Can you work these out from the drawing? Everything is in mm from the part's minimum corner. A direction names the side the tool comes from. Give positions to 0.01 mm unless a question says otherwise; leave off trailing zeros. Loops run counter-clockwise (first coordinate to the right, second up) from the corner with the lowest first, then second, coordinate; pieces in that order, holes last.
Q1. If we section it at A-A (y = 5.5): Please give me the cut outline in (x, z).
Q2. Will these pins go through, and if not, where does the flat tip stop? P1, Ø1.5, axis at x = 1.5, z = 4, coming from the -Y side; P2, Ø1, axis at y = 2, z = 7, coming from the +X side (1 decimal).
Q3. If we section it at C-C (x = 0.8): Please give me the cut outline in (y, z).
Q4. I need wall thicknesses on line 1 (Z direction, x = 2.05, y = 4.5); line 2 (X direction, y = 3.25, z = 11.25); line 3 (Y direction, x = 1.55, z = 5.5) (1 decimal). Which ranges of each line are inside material? Lowest first, please.
Q5. If we section it at B-B (z = 6.25): Please give me the cut outline in (x, y).
Q6. For the marked faces 1 and 2, which set-ups out of +Z, -Z, +X, -X, +Y, -Y let a thin tool reach every point of the face, with its end or its side?
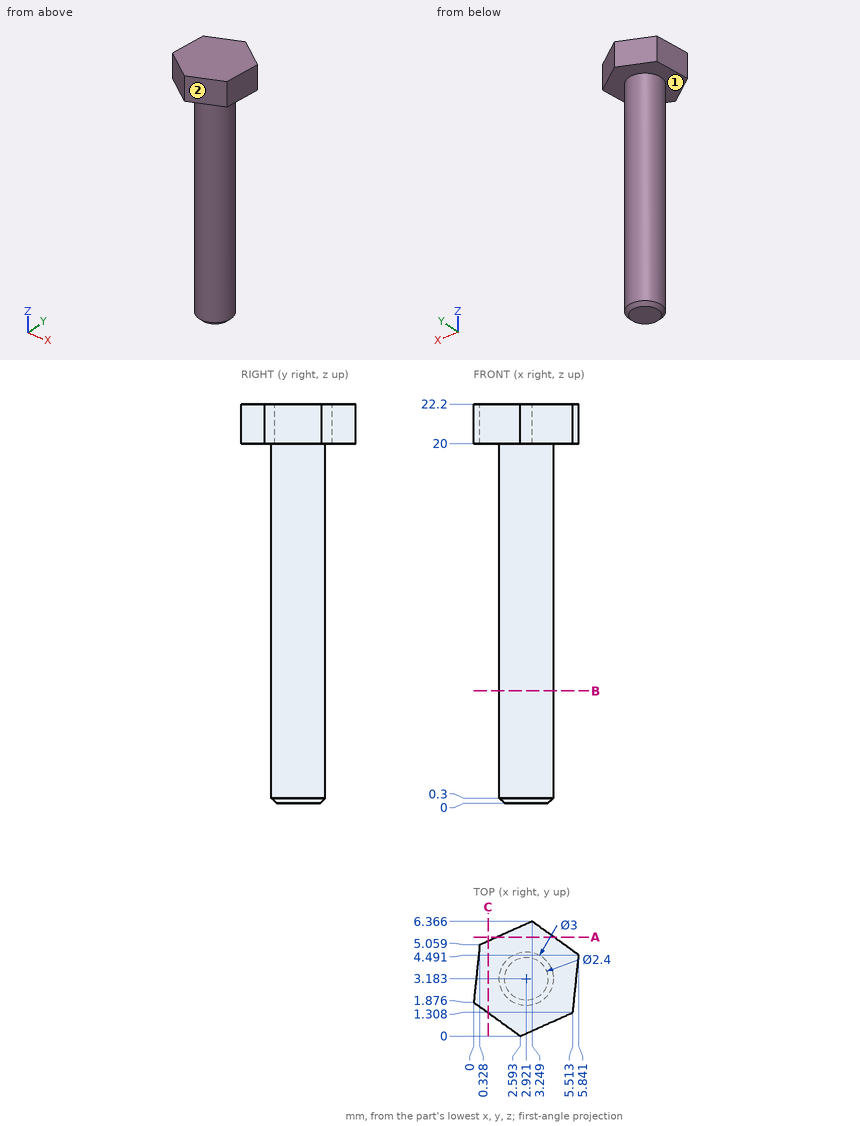
Check sheet entries:
1. outline: (1.31, 20) - (4.45, 20) - (4.45, 22.2) - (1.31, 22.2) - close
2. P1: stops at y = 1.84
2. P2: stops at x = 4.3
3. outline: (1.3, 20) - (5.27, 20) - (5.27, 22.2) - (1.3, 22.2) - close
4. line 1: z = 20 to 22.2
4. line 2: x = 1.42 to 4.42
4. line 3: y = 2.6 to 3.8
5. outline: circle Ø3 at (2.92, 3.18)
6. face 1: -Z
6. face 2: +Z, -Z, +X, -Y
